Autodesk Inventor part; units mm, degrees
ref_plane "Work Plane2" through (0, 26.25, 0) normal (0, 1, 0) x (-1, 0, 0)
ref_plane "YZ Plane" through (0, 0, 0) normal (1, 0, 0) x (0, 1, 0)
ref_plane "XY Plane" through (0, 0, 0) normal (0, 0, 1) x (1, 0, 0)
sketch "Sketch2" plane through (0, 0, 0) normal (1, 0, 0) x (0, 1, 0)
  arc A0 (15, 33.5) -> (10, 0) centre (124.725, 0) ccw construction
  arc A1 (5, 33.5) -> (0, 0) centre (114.725, 0) ccw construction
  line L0 (15, 33.5) -> (5, 33.5)
  line L1 (10, 0) -> (0, 0) construction
  line L2 (-26.4367, 0) -> (149.9186, 0)
  line L3 (10.0174, 2) -> (0.0174, 2)
  arc A2 (5, 33.5) -> (0.0174, 2) centre (114.725, 0) ccw
  arc A3 (15, 33.5) -> (10.0174, 2) centre (124.725, 0) ccw
  point P0 (0, 0)
  point P1 (15, 0)
  dimension "d6" = 5
  dimension "d8" = 10
  dimension "d10" = 10
  dimension "d12" = 2
revolve "Revolution2" add sketch "Sketch2" angle 360 about axis through (0, -10, 0) along (0, 1, 0)
ref_plane "Work Plane2" through (0, 26.25, 0) normal (0, 1, 0) x (-1, 0, 0)
sketch "Sketch5" plane through (0, 26.25, 0) normal (0, 1, 0) x (-1, 0, 0)
  circle A0 centre (0, 0) radius 33.5
  line L0 (-5.5, 33.0454) -> (5.5, 33.0454) construction
  line L1 (-5.5, 33.0454) -> (-5.5, 24.5)
  line L2 (-5.5, 24.5) -> (-3.5, 24.5)
  line L3 (-3.5, 24.5) -> (-3.5, 31.5)
  line L4 (-3.5, 31.5) -> (3.5, 31.5)
  line L5 (3.5, 31.5) -> (3.5, 24.5)
  line L6 (3.5, 24.5) -> (5.5, 24.5)
  line L7 (5.5, 24.5) -> (5.5, 33.0454)
  circle A1 centre (0, 0) radius 2
  arc A2 (5.5, 33.0454) -> (-5.5, 33.0454) centre (0, 0) ccw
  line L8 (5.5, 33.0454) -> (0, 0) construction
  line L9 (0, 0) -> (0, 33.5) construction
  line L10 (5.5, 24.5) -> (0, 0) construction
  line L11 (6.965, 32.7679) -> (0, 0) construction
  line L12 (6.965, 32.7679) -> (6.5492, 30.8116) construction
  point P0 (0, 31.5)
  dimension "d37" = 11
  dimension "d40" = 2
  dimension "d41" = 2
  dimension "d56" = 9
  dimension "d57" = 2
  dimension "d58" = 33.0454
  dimension "d59" = 2
  dimension "d60" = 0
  dimension "d61" = 0
  dimension "d62" = 12
extrude "Extrusion3" cut sketch "Sketch5" along normal through all both and the other way through all contours L7 L6 L5 L4 L3 L2 L1 A0 picked at (-4.8333, 29.6818)
sketch "Sketch6" plane through (0, 124.725, 31.5) normal (0, 0, 1) x (1, 0, 0)
  line L0 (33.5, -109.725) -> (-33.5, -109.725)
  point P0 (0, -124.725)
  point P1 (0, -114.725)
  point P2 (5.5, -109.725)
  point P3 (-5.5, -109.725)
  dimension "d45" = 5
hole "Hole2" at (0, 10, 31.5) direction (0, 0, -1) diameter 3 depth 8 tip angle 118
pattern_circular "Circular Pattern2" count 3 over 360 about axis through (0, 10, 0) along (0, 1, 0) of "Hole2", "Extrusion3"
properties part number "Parachute bulkhead" material "Plastic, Opaque White"
Read the model definition and answer for the solid it produces. Units are mm, in the model's axes. A direction names the side the tool comes from. Coordinates: 2 decimals unless noted, no trailing zeros. Write each loop counter-clockwise with the first axis right and the second up, starting at its lowest first coordinate (ties: lowest second). Pieces come first, ordered by that corner, then holes. Notation, with made-up numbers: (32, 72) - (37, 72) arc R16 ccw to (37, 94) - close; hole circle Ø6 at (20, -7.75). An arc over 180 degrees is marked (long way). Answer as a JSON object with one key per item and string values. Group by question number.
1. Each of these flat-tipped pins is pushed along its axis until it touches: P1, Ø8, axis at y = 12.5, z = 4.5, coming from the +X side; P2, Ø7.5, axis at y = 7, z = 28, coming from the +X side; P3, Ø12, axis at x = 12, z = -11, coming from the -Y side; P4, Ø5, axis at x = 0, z = 0, coming from the -Y side. Where does it stop, or does it pass through?
2. A cutting plane is placed at A-A (y = 7). Determine the outline of the cut face in (x, z).
3. Which of the six approach directions +Z, -Z, +X, -X, +Y, -Y give full straight-line access (tool end or side, diameter ignored) to faces 1 (the flat face through (5.5, 9, 29)), 2 (the flat face through (-26.915, 8.39, -16.381)), 3 (the flat face through (26.866, 8.39, -16.466)), 4 (the flat face through (22.22, 8.98, -19.18))?
4. The mould has two halves that part along Z. Classify faces 5 (the cylindrical face through (2, 5, 0)), 6 (the cylindrical face through (-0.414, 9.93, -33.497)), 7 (the flat face through (-22.12, 8.98, -19.12)), 8 (the flat face through (3.5, 9, 28)): +Z half, -Z half, draft (parallel to the pull), parting line (faces both ways), or undercut.
5. Consider L1, parallel to X at y = 10, z = 26.5; L2, parallel to Z at x = -24.5, y = 7.5; L3, parallel to Z at x = -25, y = 5.25. Determine where each line is inside the solid, lowest interval first. Write a range as [from, to].
6. A cutting plane is placed at B-B (z = 29). Give the number of separate pieces and of enclosed holes in the cut face, plus the area to 3 significant figures.
Worked out:
{
 "1": {"P1": "stops at x = 33.5", "P2": "stops at x = 23.11", "P3": "stops at y = 0.46", "P4": "stops at y = 0.02"},
 "2": {"outline": "(-31.37, -11.76) - (-23.97, -7.49) - (-22.97, -9.22) - (-29.03, -12.72) - (-25.53, -18.78) - (-19.47, -15.28) - (-18.47, -17.01) - (-25.87, -21.29) arc R33.5 ccw to (25.87, -21.29) - (18.47, -17.01) - (19.47, -15.28) - (25.53, -18.78) - (29.03, -12.72) - (22.97, -9.22) - (23.97, -7.49) - (31.37, -11.76) arc R33.5 ccw to (5.5, 33.05) - (5.5, 24.5) - (3.5, 24.5) - (3.5, 31.5) - (-3.5, 31.5) - (-3.5, 24.5) - (-5.5, 24.5) - (-5.5, 33.05) arc R33.5 ccw to start; hole circle Ø4 at (0, 0)"},
 "3": {"face 1": "+Z, +Y, -Y", "face 2": "-X, +Y, -Y", "face 3": "+X, +Y, -Y", "face 4": "+Y, -Y"},
 "4": {"face 5": "undercut", "face 6": "-Z half", "face 7": "undercut", "face 8": "draft"},
 "5": {"L1": "x = [-20.49, -5.5], [-3.5, -1.5], [1.5, 3.5], [5.5, 20.49]", "L2": "z = [-22.85, -20.5], [-18.19, -10.1], [-7.79, 22.85]", "L3": "z = [-22.3, -20.78], [-18.48, -10.39], [-8.08, 22.3]"},
 "6": {"separate pieces": "3", "enclosed holes": "1", "area": "288 mm²"}
}
